Could you check a few things on this model? Use its own coordinates, in mm. A direction names the side the tool comes from. Give positions to 0.01 mm unless a question says otherwise; leave off trailing zeros. Loops run counter-clockwise (first coordinate to the right, second up) from the corner with the lowest first, then second, coordinate; pieces in that order, holes last. Notation, with made-up numbers: M 35,68 L 82,68 A37 cw 82,104 Z; hole C -30,-23 d2. An arc over 180 degrees is marked long. Use a Markdown table: item, result. Add a question column.
1) Will these pins go through, and if not, where does the flat tip stop? pin 1 Ø5 at (x, y) = (7, -3) entering from -Z; pin 2 Ø1.1 at (y, z) = (-7.5, 0.5) entering from +X; pin 3 Ø4 at (x, z) = (8.5, 2.5) entering from -Y; pin 4 Ø2 at (x, y) = (10, -6) entering from +Z.
2) Suppose I cut it at D-D on y = -5.75. List the corners of the cut face in (x, z) for me.
3) Suppose I cut it at B-B on x = 12.75. List the corners of the cut face in (y, z) for me.
4) Suppose I cut it at C-C on z = 0.75. List the corners of the cut face in (x, y) for me.
5) We'd pull the mould along Y, two halves only. Please class faces 5 (the flat face through (18, 0, 0)), 6 (the flat face through (6, -7, 0.5)), 7 (the flat face through (3, -10, 0.5)): +Y half, -Y half, draft (parallel to the pull), parting line (faces both ways), or undercut.
6) If I drill on line 1 along Y through (x, z) = (15.25, -1.25); line 2 along Z through (x, y) = (4, -7); line 3 along X through (y, z) = (-4.75, 0.75), over which ranges is the centre line in solid material (lowest first)? Write a range as [from, to].
7) Which directions (+Z, -Z, +X, -X, +Y, -Y) give clear straight access to the entire face, cutting with the end or side of a thin tool? Please do faces 1 (the flat face through (5, -4, 0)), 2 (the flat face through (25, -2, -1)), 3 (the flat face through (6.7, -3.8, 1)), 4 (the flat face through (20, -4, 0)).
8) Suppose I cut it at A-A on y = -2. List the corners of the cut face in (x, z) for me, and give its area (3 significant figures).
Autodesk Inventor part; units mm, degrees
ref_plane "YZ Plane" through (0, 0, 0) normal (1, 0, 0) x (0, 1, 0)
ref_plane "XZ Plane" through (0, 0, 0) normal (0, 1, 0) x (-1, 0, 0)
ref_plane "XY Plane" through (0, 0, 0) normal (0, 0, 1) x (1, 0, 0)
sketch "草圖1" plane through (0, 0, 0) normal (0, 0, 1) x (1, 0, 0)
  line L0 (0, 0) -> (25, 0)
  line L1 (25, 0) -> (25, -10)
  line L2 (25, -10) -> (0, -10)
  line L3 (0, -10) -> (0, 0)
  line L4 (25, 0) -> (7, 0)
  line L5 (7, 0) -> (7, -4)
  line L6 (7, -4) -> (25, -4)
  line L7 (25, -4) -> (25, 0)
  line L8 (26, -5) -> (6, -5)
  line L9 (6, -5) -> (6, 1)
  line L10 (6, 1) -> (26, 1)
  line L11 (26, 1) -> (26, -5)
  line L12 (7, -4) -> (6, -4)
  line L13 (6, -5) -> (6, -10)
  point P0 (25, -5)
  dimension "d0" = 25
  dimension "d1" = 10
  dimension "d2" = 18
  dimension "d3" = 4
  dimension "d4" = 1
extrude "擠出1" add sketch "草圖1" along normal blind 1 contours L5 L12 L9 L0 | L0 L1 L6 L5 | L9 L13 L2 L3 L0
sketch "草圖2" plane through (0, 0, 0) normal (0, 1, 0) x (1, 0, 0)
  line L0 (25, -1) -> (0, -1)
  line L1 (25, -1) -> (24.0831, -6.2)
  line L2 (24.0831, -6.2) -> (21.9169, -6.2)
  line L3 (21.9169, -6.2) -> (17.5536, -1)
  point P0 (0, 0)
  point P1 (23, -6.2)
  dimension "d7" = 5.2
  dimension "d8" = 2
  dimension "d9" = 80
  dimension "d10" = 50
extrude "擠出2" add sketch "草圖2" against normal up to surface (4 mm away)
sketch "草圖3" plane through (0, 0, 0) normal (0, 1, 0) x (1, 0, 0)
  line L0 (25, 0) -> (0, 0)
  line L1 (0, 0) -> (0, -1)
  line L2 (17.5536, -1) -> (0, -1)
  line L3 (17.5536, -1) -> (21.9169, -6.2)
  line L4 (21.9169, -6.2) -> (24.0831, -6.2)
  line L5 (24.0831, -6.2) -> (25, -1)
  line L6 (25, 0) -> (25, -1)
  line L7 (25, 0) -> (25, 3.5)
  line L8 (25, 3.5) -> (16.5, 3.5)
  line L9 (16.5, 3.5) -> (13, 0)
  dimension "d13" = 12
  dimension "d14" = 45
  dimension "d15" = 3.5
extrude "擠出3" add sketch "草圖3" against normal up to surface (4 mm away) contours L0 L9 L8 L7
properties part number "botton_3D 列印"
Answer block:
| question | item | result |
|---|---|---|
| 1 | pin 1 | stops at z = 0 |
| 1 | pin 2 | stops at x = 6 |
| 1 | pin 3 | stops at y = -4 |
| 1 | pin 4 | passes through |
| 2 | outline | M 0,0 L 6,0 L 6,1 L 0,1 Z |
| 3 | outline | M -4,0 L 0,0 L 0,1 L -4,1 Z |
| 4 | outline | M 0,-10 L 6,-10 L 6,-4 L 25,-4 L 25,0 L 0,0 Z |
| 5 | face 5 | +Y half |
| 5 | face 6 | draft |
| 5 | face 7 | -Y half |
| 6 | line 1 | y = [-4, 0] |
| 6 | line 2 | z = [0, 1] |
| 6 | line 3 | x = [0, 6] |
| 7 | face 1 | -Z, -X, +Y, -Y |
| 7 | face 2 | +Z, -Z, +X, +Y, -Y |
| 7 | face 3 | +Z, -X, +Y, -Y |
| 7 | face 4 | +Z, -Z, +X, -Y |
| 8 | outline | M 0,0 L 13,0 L 16.5,-3.5 L 25,-3.5 L 25,1 L 24.08,6.2 L 21.92,6.2 L 17.55,1 L 0,1 Z |
| 8 | area | 85.9 mm^2 |
